The model under review builds one solid part; all positions refer to its coordinate system, in mm. Give positions to 0.01 mm unless a question says otherwise; leave off trailing zeros. Order: outer loops, then holes, each group sorted by start corner. A loop starts at its lowest first (then second) coordinate and runs counter-clockwise, first axis right, second up. Notation, with made-up numbers: M -10,49.5 L -2,49.5 A21 ccw -2,63.5 Z; hole C 79,83.25 d9. An arc over 180 degrees is marked long. One line per question, with ' | ' between items. Start each with the question number.
1. We need section B-B on x = 45.5. Write out the cut boundary in (y, z), then the cut area to 3 significant figures.
2. We need section C-C on z = 45. Write out the cut boundary in (x, y).
3. Wall thickness on L1, parallel to X at y = 314, z = 3; L2, parallel to X at y = 178, z = -24 (3 decimals); L3, parallel to Z at x = -1, y = 68: over which ranges is each line inside the solid? List them lowest first.
4. The part is to be moulded in two halves that separate along X. For faces 1 (the face through (-63.168, 225.4, -14.027)), 2 (the face through (-3.175, 232, 28)), say which applies: +X half, -X half, draft (parallel to the pull), parting line (faces both ways), or undercut.
5. Insertion check: P1, Ø6.5, axis at y = 267.5, z = 30.5, coming from the -X side; P2, Ø6.5, axis at x = 31, y = 336, coming from the -Z side; P3, Ø6.5, axis at y = 257.5, z = 30.5, coming from the +X side; P4, Ø1.5, axis at x = -48, z = 46.5, coming from the -Y side. Each pin has a flat end and moves straight along its axis. Give the tip position at first contact, or say it passes through.
```python
from build123d import *

# Parameters (mm, degrees)
SKETCH1_R           = 64.7065
SKETCH1_R_2         = 21.59
BOSS_EXTRUDE1_DEPTH = 457.2
CUT_EXTRUDE1_REACH  = 468.268
CIRPATTERN1_COUNT   = 8


with BuildPart() as part:
    # Sketch1 → Boss-Extrude1 (new body)
    with BuildSketch(Plane(origin=(0, 0, 0), x_dir=(1, 0, 0), z_dir=(0, 1, 0))):
        with Locations(Location((0, 0, 0), (0, 0, 270))):
            Circle(SKETCH1_R)
        with Locations(Location((0, 0, 0), (0, 0, 270))):
            Circle(SKETCH1_R_2, mode=Mode.SUBTRACT)
    extrude(amount=BOSS_EXTRUDE1_DEPTH)

    # Sketch2 → Cut-Extrude1 (cut, up to next)
    with BuildSketch(Plane(origin=(0, 457.2, 0), x_dir=(1, 0, 0), z_dir=(0, 1, 0)), mode=Mode.PRIVATE) as cut_extrude1_sk1:
        with BuildLine():
            Line((-3.175, 34.29), (3.175, 34.29))
            Line((3.175, 34.29), (3.175, 21.355268085))
            ThreePointArc((3.175, 21.355268085), (0, 21.59), (-3.175, 21.355268085))
            Line((-3.175, 21.355268085), (-3.175, 34.29))
        make_face()
    cut_extrude1_tool1 = extrude(cut_extrude1_sk1.sketch, amount=-CUT_EXTRUDE1_REACH, mode=Mode.PRIVATE) & part.part
    cut_extrude1 = cut_extrude1_tool1.solids().sort_by_distance((0, 457.2, -27.900772))[0]
    add(cut_extrude1, mode=Mode.SUBTRACT)

    # CirPattern1: Cut-Extrude1 ×8 about axis
    cirpattern1_axis = Axis((0, 0, 0), (0, 1, 0))
    for i in range(1, CIRPATTERN1_COUNT):
        add(cut_extrude1.rotate(cirpattern1_axis, i * 360 / CIRPATTERN1_COUNT), mode=Mode.SUBTRACT)


solid = part.part
```
Entries:
1) outline: M 0,-46.01 L 457.2,-46.01 L 457.2,46.01 L 0,46.01 Z | area: 42,100 mm^2
2) outline: M -46.5,0 L 46.5,0 L 46.5,457.2 L -46.5,457.2 Z
3) L1: x = -64.64 to -34.29, 34.29 to 64.64 | L2: x = -60.091 to -24.493, -19.51 to -3.175, 3.175 to 19.51, 24.493 to 60.091 | L3: z = -64.7 to -34.29, 34.29 to 64.7
4) face 1: parting line | face 2: undercut
5) P1: stops at x = -58.69 | P2: stops at z = -58.45 | P3: stops at x = 58.69 | P4: passes through
